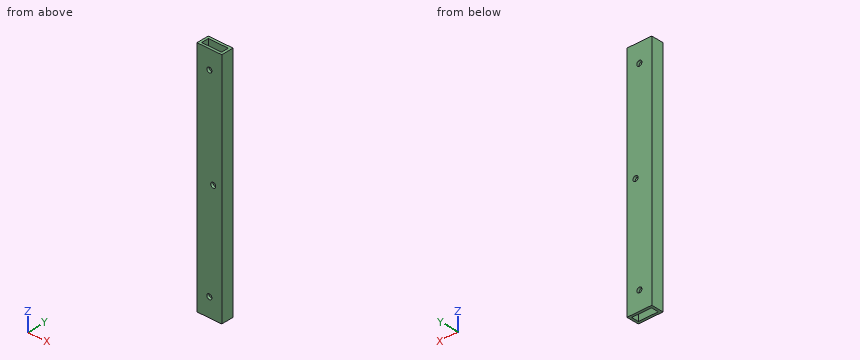
from build123d import *

# Parameters (mm, degrees)
SKETCH_1_W          = 20
SKETCH_1_H          = 10
SKETCH_1_W_2        = 16
SKETCH_1_H_2        = 6
EXTRUDE_1_DEPTH     = 95
SKETCH_3_R          = 2.05
CUT_EXTRUDE_1_DEPTH = 97.050697163


with BuildPart() as part:
    # 草图1 → 凸台-拉伸1 (new, symmetric)
    with BuildSketch(Plane.XY):
        with Locations((0.036753729, 0.03823935)):
            Rectangle(SKETCH_1_W, SKETCH_1_H)
        with Locations((0.036753729, 0.03823935)):
            Rectangle(SKETCH_1_W_2, SKETCH_1_H_2, mode=Mode.SUBTRACT)
    extrude(amount=EXTRUDE_1_DEPTH, both=True)

    # 草图3 → 切除-拉伸1 (cut, through all)
    with BuildSketch(Plane(origin=(0, 5.03823935, 0), x_dir=(1, 0, 0), z_dir=(0, 1, 0))):
        with Locations(Location((3.136753729, 0, 0), (0, 0, 270))):
            Circle(SKETCH_3_R)
        with Locations(Location((0.036753729, 80, 0), (0, 0, 270))):
            Circle(SKETCH_3_R)
        with Locations(Location((0.036753729, -80, 0), (0, 0, 270))):
            Circle(SKETCH_3_R)
    extrude(amount=-CUT_EXTRUDE_1_DEPTH, mode=Mode.SUBTRACT)


solid = part.part
The listing builds one solid part. Answer for the finished solid, in the listing's coordinates (mm). Give positions to 0.01 mm unless a question says otherwise; leave off trailing zeros. Write each loop counter-clockwise with the first axis right and the second up, starting at its lowest first coordinate (ties: lowest second). Pieces come first, ordered by that corner, then holes.
1) Section A-A (z = 6.5) is taken. Write down the section's boundary in (x, y).
2) Section B-B (z = -80) is taken. Write down the section's boundary in (x, y), and give its area (3 significant figures).
3) Find the intervals of material crossed by L1, parallel to X at y = -1, z = -19.5; L2, parallel to X at y = 4, z = 80; L3, parallel to Y at x = -0.75, z = -43, in increasing order.
Response:
1. outline: (-9.96, -4.96) - (10.04, -4.96) - (10.04, 5.04) - (-9.96, 5.04) - close; hole (-7.96, -2.96) - (8.04, -2.96) - (8.04, 3.04) - (-7.96, 3.04) - close
2. outline: (-9.96, -4.96) - (-2.01, -4.96) - (-2.01, -2.96) - (-7.96, -2.96) - (-7.96, 3.04) - (-2.01, 3.04) - (-2.01, 5.04) - (-9.96, 5.04) - close; (2.09, -4.96) - (10.04, -4.96) - (10.04, 5.04) - (2.09, 5.04) - (2.09, 3.04) - (8.04, 3.04) - (8.04, -2.96) - (2.09, -2.96) - close
2. area: 87.6 mm2
3. L1: x = -9.96 to -7.96, 8.04 to 10.04
3. L2: x = -9.96 to -2.01, 2.09 to 10.04
3. L3: y = -4.96 to -2.96, 3.04 to 5.04
